Here's how the part is built. I have some questions about the finished solid (model axes, mm). A direction names the side the tool comes from. Round coordinates to 2 decimals unless told otherwise and drop trailing zeros. Write each loop counter-clockwise with the first axis right and the second up, starting at its lowest first coordinate (ties: lowest second). Pieces come first, ordered by that corner, then holes. Notation, with made-up numbers: (33, -13) - (55, -13) arc R18 cw to (55, 22) - close; hole circle Ø8 at (26.25, -37). An arc over 180 degrees is marked (long way). Return JSON: item names as keys, results as strings. Group by question number.
```python
from build123d import *

# Parameters (mm, degrees)
F0_R     = 2.54
F1_DEPTH = 1.524
F2_R     = 2.54
F2_R_2   = 6.35
F3_DEPTH = 0.254
F4_R     = 3.175
F5_DEPTH = 12.7


with BuildPart() as f1:
    # F0 (on Top) → F1 (new body)
    with BuildSketch(Plane.XY):
        with BuildLine():
            ThreePointArc((-18.383103, -12.44771), (-17.862339, -13.704946), (-16.605103, -14.22571))
            Line((-16.605103, -14.22571), (113.188897, -14.22571))
            ThreePointArc((113.188897, -14.22571), (114.446133, -13.704946), (114.966897, -12.44771))
            Line((114.966897, -12.44771), (114.966897, 52.32229))
            ThreePointArc((114.966897, 52.32229), (114.446133, 53.579526), (113.188897, 54.10029))
            Line((113.188897, 54.10029), (-16.605103, 54.10029))
            ThreePointArc((-16.605103, 54.10029), (-17.862339, 53.579526), (-18.383103, 52.32229))
            Line((-18.383103, 52.32229), (-18.383103, -12.44771))
        make_face()
        with Locations((5.623456, -8.63771)):
            Circle(F0_R, mode=Mode.SUBTRACT)
        with Locations((69.123456, -8.63771)):
            Circle(F0_R, mode=Mode.SUBTRACT)
        with Locations((8.518225, 48.51229)):
            Circle(F0_R, mode=Mode.SUBTRACT)
        with Locations((72.018225, 48.51229)):
            Circle(F0_R, mode=Mode.SUBTRACT)
    extrude(amount=F1_DEPTH)

    # F2 (on face) → F3 (join)
    with BuildSketch(Plane.XY.offset(1.524)):
        with BuildLine():
            Line((-18.383103, 52.32229), (-18.383103, -12.44771))
            ThreePointArc((-18.383103, -12.44771), (-17.862339, -13.704946), (-16.605103, -14.22571))
            Line((-16.605103, -14.22571), (113.188897, -14.22571))
            ThreePointArc((113.188897, -14.22571), (114.446133, -13.704946), (114.966897, -12.44771))
            Line((114.966897, -12.44771), (114.966897, 52.32229))
            ThreePointArc((114.966897, 52.32229), (114.446133, 53.579526), (113.188897, 54.10029))
            Line((113.188897, 54.10029), (-16.605103, 54.10029))
            ThreePointArc((-16.605103, 54.10029), (-17.862339, 53.579526), (-18.383103, 52.32229))
        make_face()
        with Locations((5.623456, -8.63771)):
            Circle(F2_R, mode=Mode.SUBTRACT)
        with Locations((69.123456, -8.63771)):
            Circle(F2_R, mode=Mode.SUBTRACT)
        with Locations((8.518225, 48.51229)):
            Circle(F2_R, mode=Mode.SUBTRACT)
        with Locations((95.916897, 35.05029)):
            Circle(F2_R_2, mode=Mode.SUBTRACT)
        with Locations((72.018225, 48.51229)):
            Circle(F2_R, mode=Mode.SUBTRACT)
    extrude(amount=F3_DEPTH)

    # F4 (on face) → F5 (join)
    with BuildSketch(Plane.XY.offset(1.524)):
        with Locations((95.916897, 35.05029)):
            Circle(F4_R)
    extrude(amount=F5_DEPTH)


solid = f1.part
```
1) If we mould it in two halves opening along Y, with no side actions, what happens to faces 3 (the flat face through (96, 35, 14.224)), 4 (the cylindrical face through (7.968, 46.033, 0.877))? For each: released by +Y, released by -Y, zero draft, split by the parting line, or undercut.
2) Imagine slicing it at C-C (x = 54.5). Please give me the cut outline in (y, z).
3) Imagine slicing it at B-B (y = 21.5). Please give me the cut outline in (x, z), plus the area to 3 significant figures.
4) Imagine slicing it at A-A (x = 9.5). Please give me the cut outline in (y, z), plus the area to 3 significant figures.
5) I need wall thicknesses on line 1 along Z through (x, y) = (22, 49.5). Which ranges of the line are inside material? Lowest first, please.
6) Imagine slicing it at D-D (z = 5.75). Please give me the cut outline in (x, y) (3 decimals), plus the area to 3 significant figures.
7) For faces 1 (the flat face through (93, 37, 1.524)), 2 (the cylindrical face through (7.97, -9.61, 0.88)), which set-ups out of +Z, -Z, +X, -X, +Y, -Y let a thin tool reach every point of the face, with its end or its side?
8) Will these pins go through, and if not, where does the flat tip stop? pin 1 Ø20.5 at (x, y) = (22.5, 20.5) entering from +Z; pin 2 Ø6 at (x, y) = (76.5, 1.5) entering from -Z; pin 3 Ø2 at (y, z) = (45.5, 3.5) entering from +X; pin 4 Ø8 at (y, z) = (28.5, 12.5) entering from +X.
Results found:
{
 "1": {"face 3": "zero draft", "face 4": "undercut"},
 "2": {"outline": "(-14.23, 0) - (54.1, 0) - (54.1, 1.78) - (-14.23, 1.78) - close"},
 "3": {"outline": "(-18.38, 0) - (114.97, 0) - (114.97, 1.78) - (-18.38, 1.78) - close", "area": "237 mm²"},
 "4": {"outline": "(-14.23, 0) - (46.17, 0) - (46.17, 1.78) - (-14.23, 1.78) - close; (50.85, 0) - (54.1, 0) - (54.1, 1.78) - (50.85, 1.78) - close", "area": "113 mm²"},
 "5": {"line 1": "z = 0 to 1.78"},
 "6": {"outline": "circle Ø6.35 at (95.917, 35.05)", "area": "31.7 mm²"},
 "7": {"face 1": "+Z", "face 2": "+Z, -Z"},
 "8": {"pin 1": "stops at z = 1.78", "pin 2": "stops at z = 0", "pin 3": "passes through", "pin 4": "stops at x = 97.81"}
}
